Autodesk Inventor part; units mm, degrees
ref_plane "YZ Plane" through (0, 0, 0) normal (1, 0, 0) x (0, 1, 0)
ref_plane "XZ Plane" through (0, 0, 0) normal (0, 1, 0) x (-1, 0, 0)
ref_plane "XY Plane" through (0, 0, 0) normal (0, 0, 1) x (1, 0, 0)
sketch "Sketch1" plane through (0, 0, 0) normal (0, 0, 1) x (1, 0, 0)
  line L0 (-14.2875, 41.656) -> (14.2875, 41.656)
  line L1 (14.2875, 41.656) -> (14.2875, -41.656)
  line L2 (14.2875, -41.656) -> (-14.2875, -41.656)
  line L3 (-14.2875, -41.656) -> (-14.2875, 41.656)
  point P0 (0, 0)
  dimension "d0" = 28.575
  dimension "d1" = 83.312
  dimension "d2" = 14.2875
  dimension "d3" = 41.656
extrude "Plate2" add sketch "Sketch1" along normal blind 3.048
sketch "Sketch2" plane through (-14.2875, 38.608, 0) normal (0, 1, 0) x (-1, 0, 0)
  line L0 (-28.575, 0) -> (0, 0)
  line L1 (0, 0) -> (0, 12.573)
  line L2 (0, 12.573) -> (-28.575, 12.573)
  line L3 (-28.575, 12.573) -> (-28.575, 0)
edge flange "Flange1" height 9.525 angle 90 thickness 3.048 bend radius 3.048 thickness toward (0, 1, 0) relief tear relief width 3.048 relief depth 1.524 corner gap 3.048 corner form 0 edges at (0, 41.656, 3.048) (0, -41.656, 3.048) wall of the first edge with corners at (14.2875, 38.608, 0) (-14.2875, 38.608, 0) (-14.2875, 38.608, 12.573) (14.2875, 38.608, 12.573)
bend "Bend1"
corner "Corner1"
sketch "Sketch3" plane through (-14.2875, -38.608, 12.573) normal (0, 1, 0) x (1, 0, 0)
  line L0 (0, 0) -> (0, 6.477)
  line L1 (0, 0) -> (28.575, 0)
  line L2 (28.575, 0) -> (28.575, 6.477)
  point P0 (14.2875, 12.573)
  point P1 (3.175, 3.175)
  point P2 (25.4, 3.175)
  dimension "d16" = 3.175
  dimension "d17" = 3.175
  dimension "d18" = 3.175
  dimension "d19" = 3.175
hole "Hole1" at (-11.1125, -38.608, 9.398) at (11.1125, -38.608, 9.398) direction (0, -1, 0) diameter 3.175 end through all
sketch "Sketch5" plane through (-14.2875, 41.656, 12.573) normal (0, 1, 0) x (1, 0, 0)
  circle A0 centre (3.175, 3.175) radius 1.5875
  circle A1 centre (25.4, 3.175) radius 1.5875
  point P0 (14.2875, 12.573)
hole "Hole2" at (-11.1125, 41.656, 9.398) at (11.1125, 41.656, 9.398) direction (0, -1, 0) diameter 3.175 end through all
equation "\"d25\" = Thickness"
equation "\"d32\" = Thickness"
equation "\"d6\" = BendReliefWidth"
equation "\"d7\" = BendReliefDepth"
equation "\"d8\" = MinimumRemnant"
equation "\"d9\" = BendRadius"
equation "\"d12\" = BendRadius"
equation "\"d13\" = CornerReliefSize"
equation "\"d14\" = GapSize"
equation "\"d15\" = JacobiRadiusSize"
equation "\"BendRadius\" = Thickness"
equation "\"BendReliefWidth\" = Thickness"
equation "\"BendReliefDepth\" = 0.5 * Thickness"
equation "\"CornerReliefSize\" = 4 * Thickness"
equation "\"MinimumRemnant\" = 2 * Thickness"
equation "\"TransitionRadius\" = BendRadius"
equation "\"JacobiRadiusSize\" = BendRadius"
equation "\"GapSize\" = Thickness"
equation "\"d4\" = BendRadius"
equation "\"d5\" = BendRadius"
properties part number "gearbox rib"
Can you work these out from the model? Positions are in its coordinate system, mm. A direction names the side the tool comes from. Coordinates: 2 decimals unless noted, no trailing zeros. Loops run counter-clockwise (first coordinate to the right, second up) from the corner with the lowest first, then second, coordinate; pieces in that order, holes last. Notation, with made-up numbers: M 37,37.25 L 58,37.25 A14 cw 58,49.25 Z; hole C 85.5,-35 d3. An arc over 180 degrees is marked long. Return JSON: item names as keys, results as strings. Group by question number.
Item 1: Imagine slicing it at B-B (x = -8). Please give me the cut outline in (y, z).
Item 2: On a 3-axis mill with a long thin cutter (end or side, diameter ignored), from which of +Z, -Z, +X, -X, +Y, -Y can I reach the whole of each face in a straight line? I mean faces 1 (the flat face through (0, 41.656, 9)), 2 (the cylindrical face through (0.2, -37.739, 3.965)). Say none if no direction works.
Item 3: Imagine slicing it at C-C (z = 9.25). Please give me the cut outline in (x, y), and give its area (3 significant figures).
Item 4: Imagine slicing it at A-A (z = 4.5). Please give me the cut outline in (x, y).
Item 5: If I drill on L1, parallel to Y at x = -8, z = 9; L2, parallel to Z at x = -4.25, y = -11; L3, parallel to Y at x = 0.25, z = 4, over which ranges is the centre line in solid material (lowest first)? Write a range as from..to.
Item 6: Thinking about a two-plate mould opening in Z: for faces 3 (the flat face through (-14.288, 0.2, 2.6)), 4 (the cylindrical face through (-11.59, 40.11, 10.91)), 5 (the cylindrical face through (-0.2, 37.739, 3.965)), which applies, released by +Z, released by -Z, zero draft, split by the parting line, or undercut?
Item 7: Imagine slicing it at D-D (y = -33.5). Please give me the cut outline in (x, z), and give its area (3 significant figures).
Item 8: I'm going to push a flat-ended pin straight in: pin 1 Ø5 at (x, y) = (-9, -18.5) entering from +Z. Where does the tip first touch, or does it pass through?
Verdict:
{
 "1": {"outline": "M -41.66,6.1 A6.1 ccw -35.56,0 L 35.56,0 A6.1 ccw 41.66,6.1 L 41.66,12.57 L 38.61,12.57 L 38.61,6.1 A3.05 cw 35.56,3.05 L -35.56,3.05 A3.05 cw -38.61,6.1 L -38.61,12.57 L -41.66,12.57 Z"},
 "2": {"face 1": "+Z, -Z, +X, -X, +Y", "face 2": "+Z, +X, -X"},
 "3": {"outline": "M -14.29,-41.66 L -12.69,-41.66 L -12.69,-38.61 L -14.29,-38.61 Z; M -14.29,38.61 L -12.69,38.61 L -12.69,41.66 L -14.29,41.66 Z; M -9.53,-41.66 L 9.53,-41.66 L 9.53,-38.61 L -9.53,-38.61 Z; M -9.53,38.61 L 9.53,38.61 L 9.53,41.66 L -9.53,41.66 Z; M 12.69,-41.66 L 14.29,-41.66 L 14.29,-38.61 L 12.69,-38.61 Z; M 12.69,38.61 L 14.29,38.61 L 14.29,41.66 L 12.69,41.66 Z", "area": "136 mm^2"},
 "4": {"outline": "M -14.29,-41.44 L 14.29,-41.44 L 14.29,-38.16 L -14.29,-38.16 Z; M -14.29,38.16 L 14.29,38.16 L 14.29,41.44 L -14.29,41.44 Z"},
 "5": {"L1": "y = -41.66..-38.61, 38.61..41.66", "L2": "z = 0..3.05", "L3": "y = -41.28..-37.77, 37.77..41.28"},
 "6": {"face 3": "zero draft", "face 4": "undercut", "face 5": "released by +Z"},
 "7": {"outline": "M -14.29,0 L 14.29,0 L 14.29,3.05 L -14.29,3.05 Z", "area": "87.1 mm^2"},
 "8": {"pin 1": "stops at z = 3.05"}
}
